Geometry: final body of the model. Coordinates: model frame, mm. Face numbers are marked on the shaded views. A direction names the side the tool comes from. Give positions to 0.01 mm unless a question says otherwise; leave off trailing zeros. Write each loop counter-clockwise with the first axis right and the second up, starting at its lowest first coordinate (ties: lowest second). Pieces come first, ordered by that corner, then holes. Notation, with made-up numbers: (69, 6) -> (89, 6) arc R12 cw to (89, 12) -> close; hole circle Ø1 at (-39.75, 8.25). An arc over 180 degrees is marked (long way). Use CSV: the item, a comma, the result in double quotes. Start each with the question number.
1) Draft query along Z for the marked faces 4, 5 and 6. Return one class per face: pulls with the +Z half, pulls with the -Z half, needs draft (parallel to the pull), parting line crosses it, or undercut.
2) Material intervals for line 1 (Y direction, x = -13, z = -10.5) (3 decimals); line 2 (Z direction, x = -7.25, y = 13) (3 decimals); line 3 (Y direction, x = -22.5, z = -18.5), sorted ascending. Write a range as [from, to].
3) Section C-C (y = 9). Output: boundary loops of the cut face in (x, z) (3 decimals), plus the area to 3 significant figures.
4) Set-up query: the marked faces 1, 2 and 3. Return all of +Z, -Z, +X, -X, +Y, -Y with unobstructed straight access to the full face (end or side cutting, diameter ignored); none if empty.
5) Section B-B (x = -12.5). Output: boundary loops of the cut face in (y, z) (1 decimal), plus the area to 3 significant figures.
6) Section D-D (z = -13.75). Output: boundary loops of the cut face in (x, y) (3 decimals).
7) Contact query for flat-ended pins moving along their axis: P1, Ø8, axis at x = -11, y = 20.5, coming from the +Z side (3 decimals); P2, Ø6, axis at y = 10, z = -14, coming from the +X side; P3, Ø5, axis at x = -7, z = -9, coming from the +Y side (3 decimals); P4, Ø1, axis at x = -26.5, y = 1.5, coming from the -Z side. Output: stop coordinate, or through.
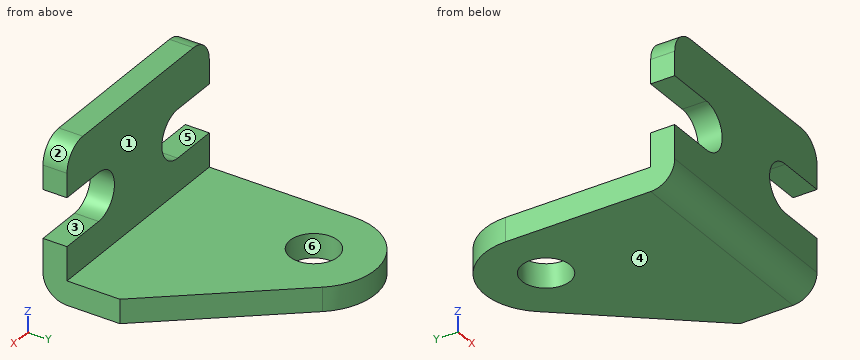
Autodesk Inventor part; units mm, degrees
ref_plane "YZ Plane" through (0, 0, 0) normal (1, 0, 0) x (0, 1, 0)
ref_plane "XZ Plane" through (0, 0, 0) normal (0, 1, 0) x (-1, 0, 0)
ref_plane "XY Plane" through (0, 0, 0) normal (0, 0, 1) x (1, 0, 0)
sketch "Sketch1" plane through (0, 0, 0) normal (0, 1, 0) x (-1, 0, 0)
  line L0 (0, 0) -> (28.575, 0)
  line L1 (28.575, 0) -> (28.575, -20.32)
  line L2 (28.575, -20.32) -> (0, -20.32)
  line L3 (0, -20.32) -> (0, 0)
  dimension "d0" = 28.575
  dimension "d1" = 20.32
extrude "Extrusion1" add sketch "Sketch1" along normal blind 3.175
fillet "Fillet1" radius 3.175 1 edges at (-14.2875, 0, -20.32)
fillet "Fillet2" radius 3.175 1 edges at (0, 1.5875, 0)
fillet "Fillet3" radius 3.175 1 edges at (-28.575, 1.5875, 0)
sketch "Sketch2" plane through (0, 3.175, 0) normal (0, 1, 0) x (1, 0, 0)
  line L0 (-28.575, 20.32) -> (-28.575, 3.175)
  line L1 (0, 3.175) -> (0, 20.32)
  line L2 (-28.575, 20.32) -> (0, 20.32)
  line L3 (0, 20.32) -> (0, 17.145)
  line L4 (0, 17.145) -> (-28.575, 17.145)
  line L5 (-28.575, 17.145) -> (-28.575, 20.32)
  point P0 (0, 0)
  dimension "d7" = 3.175
extrude "Extrusion2" add sketch "Sketch2" along normal blind 6.985
sketch "Sketch3" plane through (0, 3.175, 0) normal (0, 1, 0) x (1, 0, 0)
  line L0 (0, 17.145) -> (0, 3.175)
  line L1 (0, 6.35) -> (-6.35, 6.35)
  line L2 (-6.35, 6.35) -> (-6.35, 12.7)
  line L3 (-6.35, 12.7) -> (0, 12.7)
  line L4 (0, 12.7) -> (0, 6.35)
  line L5 (-28.575, 3.175) -> (-28.575, 17.145)
  line L6 (-28.575, 6.35) -> (-22.225, 6.35)
  line L7 (-22.225, 6.35) -> (-22.225, 12.7)
  line L8 (-22.225, 12.7) -> (-28.575, 12.7)
  line L9 (-28.575, 12.7) -> (-28.575, 6.35)
  line L10 (-25.4, 0) -> (-3.175, 0)
  line L11 (0, 20.32) -> (-28.575, 20.32)
  circle A0 centre (-6.35, 9.525) radius 3.175
  circle A1 centre (-22.225, 9.525) radius 3.175
  point P0 (0, 0)
  dimension "d10" = 6.35
  dimension "d11" = 7.62
  dimension "d12" = 6.35
  dimension "d13" = 6.35
extrude "Extrusion3" cut sketch "Sketch3" against normal blind 25.4
sketch "Sketch4" plane through (-28.575, 3.175, -17.145) normal (0, 0, 1) x (1, 0, 0)
  line L0 (0, 0) -> (0, 6.985)
  line L1 (0, 6.985) -> (28.4507, 6.985)
  line L2 (28.575, 0) -> (0, 0)
  line L3 (28.575, -3.175) -> (0, -3.175)
  dimension "d16" = 6.985
  dimension "d17" = 10.16
sketch "Sketch5" plane through (-28.575, 3.175, -17.145) normal (0, 0, 1) x (1, 0, 0)
  line L0 (28.575, 0) -> (28.575, 6.985)
  line L1 (28.575, 6.985) -> (0, 41.275)
  line L2 (28.575, -3.175) -> (0, -3.175)
  line L3 (0, 0) -> (0, 6.985)
  line L4 (28.575, 0) -> (0, 0)
  line L5 (0, 41.275) -> (0, 6.985)
  line L6 (0, 0) -> (0, 6.985)
  line L7 (0, 6.985) -> (28.575, 6.985)
  dimension "d18" = 44.45
  dimension "d19" = 0
  dimension "d20" = 6.985
  dimension "d21" = 6.985
extrude "Extrusion4" add sketch "Sketch5" against normal blind 3.175 contours L7 L5 L1
sketch "Sketch6" plane through (-28.575, 3.175, -17.145) normal (0, 0, 1) x (1, 0, 0)
  circle A0 centre (7.9375, 19.05) radius 3.175
  line L0 (28.575, -3.175) -> (0, -3.175)
  line L1 (0, 0) -> (0, 41.275)
  dimension "d24" = 22.225
  dimension "d25" = 7.9375
  dimension "d26" = 6.35
extrude "Extrusion5" cut sketch "Sketch6" against normal blind 3.175
sketch "Sketch7" plane through (-28.575, 3.175, -17.145) normal (0, 0, 1) x (1, 0, 0)
  line L0 (0, 0) -> (0, 41.275)
  line L1 (28.575, 6.985) -> (0, 41.275)
  circle A0 centre (7.9375, 19.05) radius 3.175
  point P0 (28.575, -3.175)
fillet "Fillet4" radius 8.001 1 edges at (-28.575, 44.45, -18.7325)
properties part number "LeftPinAtttachments-1111-2019"
Answers follow:
1,face 4,"pulls with the -Z half"
1,face 5,"undercut"
1,face 6,"needs draft"
2,line 1,"y = [0, 3.175]"
2,line 2,"z = [-20.32, -17.145]"
2,line 3,"y = [0.3, 19.65], [24.8, 30.12]"
3,outline,"(-28.575, -20.32) -> (0, -20.32) -> (0, -17.145) -> (-28.575, -17.145) -> close"
3,area,"90.7 mm^2"
4,face 1,"+Z, +X, -X, +Y"
4,face 2,"+Z, +X, +Y, -Y"
4,face 3,"+X, +Y, -Y"
5,outline,"(0, -17.1) arc R3.2 ccw to (3.2, -20.3) -> (25.2, -20.3) -> (25.2, -17.1) -> (3.2, -17.1) -> (3.2, 0) -> (0, 0) -> close"
5,area,"132 mm^2"
6,outline,"(-28.575, 0) -> (0, 0) -> (0, 3.175) -> (-28.575, 3.175) -> close"
7,P1,"stops at z = -17.145"
7,P2,"passes through"
7,P3,"stops at y = 3.175"
7,P4,"stops at z = -20.09"
